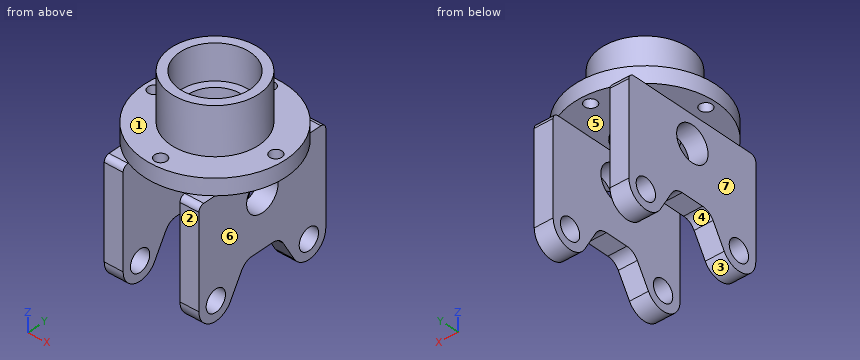
from build123d import *

# Parameters (mm, degrees)
SKETCH_1_R               = 52.5
EXTRUDE_1_DEPTH          = 12
SKETCH_2_R               = 32.5
EXTRUDE_2_DEPTH          = 35
SKETCH_3_R               = 26
CUT_EXTRUDE_1_DEPTH      = 26
SKETCH_4_R               = 20
CUT_EXTRUDE_2_DEPTH      = 21
SKETCH_5_R               = 8
SKETCH_5_R_2             = 13
EXTRUDE_3_DEPTH          = 35
SKETCH_6_W               = 42
SKETCH_6_H               = 101.243911614
CUT_EXTRUDE_3_DEPTH      = 153.922365925
SKETCH_7_R               = 4.5
CUT_EXTRUDE_4_DEPTH      = 114.615579918
PATTERN_CIRCULAR_1_COUNT = 4


with BuildPart() as part:
    # 草图1 → 凸台-拉伸1 (new body)
    with BuildSketch(Plane.XY):
        Circle(SKETCH_1_R)
    extrude(amount=-EXTRUDE_1_DEPTH)

    # 草图2 → 凸台-拉伸2 (add)
    with BuildSketch(Plane.XY):
        Circle(SKETCH_2_R)
    extrude(amount=EXTRUDE_2_DEPTH)

    # 草图3 → 切除-拉伸1 (cut)
    with BuildSketch(Plane.XY.offset(35)):
        Circle(SKETCH_3_R)
    extrude(amount=-CUT_EXTRUDE_1_DEPTH, mode=Mode.SUBTRACT)

    # 草图4 → 切除-拉伸2 (cut)
    with BuildSketch(Plane.XY.offset(9)):
        Circle(SKETCH_4_R)
    extrude(amount=-CUT_EXTRUDE_2_DEPTH, mode=Mode.SUBTRACT)

    # 草图5 → 凸台-拉伸3 (add, symmetric)
    with BuildSketch(Plane(origin=(0, 0, 0), x_dir=(0, 0, -1), z_dir=(1, 0, 0))):
        with BuildLine():
            Line((84, -52.5), (16, -52.5))
            ThreePointArc((16, -52.5), (13.171572875, -51.328427125), (12, -48.5))
            Line((12, -48.5), (12, 48.5))
            ThreePointArc((12, 48.5), (13.171572875, 51.328427125), (16, 52.5))
            Line((16, 52.5), (84, 52.5))
            ThreePointArc((84, 52.5), (97.522961568, 42.123466631), (91, 26.375644347))
            Line((91, 26.375644347), (75, 17.13804004))
            ThreePointArc((75, 17.13804004), (71.339745962, 13.477786002), (70, 8.477786002))
            Line((70, 8.477786002), (70, -8.477786002))
            ThreePointArc((70, -8.477786002), (71.339745962, -13.477786002), (75, -17.13804004))
            Line((75, -17.13804004), (91, -26.375644347))
            ThreePointArc((91, -26.375644347), (97.522961568, -42.123466631), (84, -52.5))
        make_face()
        with Locations((84, 38.5)):
            Circle(SKETCH_5_R, mode=Mode.SUBTRACT)
        with Locations((84, -38.5)):
            Circle(SKETCH_5_R, mode=Mode.SUBTRACT)
        with Locations((32, 0)):
            Circle(SKETCH_5_R_2, mode=Mode.SUBTRACT)
    extrude(amount=EXTRUDE_3_DEPTH, both=True)

    # 草图6 → 切除-拉伸3 (cut, through all)
    with BuildSketch(Plane.XZ.offset(52.5)):
        with Locations((0, -62.621955807)):
            Rectangle(SKETCH_6_W, SKETCH_6_H)
    extrude(amount=-CUT_EXTRUDE_3_DEPTH, mode=Mode.SUBTRACT)

    # 草图7 → 切除-拉伸4 (cut, through all)
    with BuildSketch(Plane(origin=(0, 0, -12), x_dir=(-1, 0, 0), z_dir=(0, 0, -1))):
        with Locations((-45, 0)):
            Circle(SKETCH_7_R)
    cut_extrude_4 = extrude(amount=-CUT_EXTRUDE_4_DEPTH, mode=Mode.SUBTRACT)

    # 阵列(圆周)1: 切除-拉伸4 ×4 about axis
    pattern_circular_1_axis = Axis((0, 0, 0), (0, 0, 1))
    for i in range(1, PATTERN_CIRCULAR_1_COUNT):
        add(cut_extrude_4.rotate(pattern_circular_1_axis, i * 360 / PATTERN_CIRCULAR_1_COUNT), mode=Mode.SUBTRACT)


solid = part.part
Build history of the part. All positions in model axes, mm. Face numbers are marked on the shaded views. A direction names the side the tool comes from. Give positions to 0.01 mm unless a question says otherwise; leave off trailing zeros. Write each loop counter-clockwise with the first axis right and the second up, starting at its lowest first coordinate (ties: lowest second). Pieces come first, ordered by that corner, then holes. Notation, with made-up numbers: (2.5, -25.75) - (21.5, -25.75) arc R34 ccw to (21.5, 4.25) - close; hole circle Ø4 at (55.25, 79). An arc over 180 degrees is marked (long way). Use one line per item in the form item = value. Start each with the question number.
1. Band-saw the part on C-C on y = 43. Write the cut outline in (x, z), plus the area to 3 significant figures.
2. 3-axis set-ups, long thin cutter, end or side, ignore diameter. For the marked faces 4, 5, 6 and 7: which of +Z, -Z, +X, -X, +Y, -Y reach the whole face in a straight line?
3. Band-saw the part on D-D on x = -45. Write the cut outline in (y, z).
4. Two-plate mould, pull along Y, no slides. Class the marked faces 1, 2 and 3: released by +Y, released by -Y, zero draft, split by the parting line, or undercut.
5. Drop flat-ended pins along their axis: pin 1 Ø1 at (x, y) = (40, -16.5) entering from +Z; pin 2 Ø8 at (x, y) = (-19.5, -21) entering from -Z; pin 3 Ø7 at (x, y) = (-26.5, -1) entering from -Z; pin 4 Ø12 at (x, z) = (19.5, -80.5) entering from -Y. Give the stop position or say it passes through.
6. Band-saw the part on B-B on x = 0. Write the cut outline in (y, z), plus the area to 3 significant figures.
7. Band-saw the part on A-A on z = -32. Write the cut outline in (x, y).
8. Probe line 1 (Y direction, x = 0, z = 23.75); line 2 (Z direction, x = -28, y = 1); line 3 (Y direction, x = -31.5, z = -84). List the from-to ranges inside material, lowest first. Write a range as [from, to].
Conclusion:
q1.outline = (-35, -97.26) - (-21, -97.26) - (-21, -90.61) - (-35, -90.61) - close; (-35, -77.39) - (-21, -77.39) - (-21, -12) - (-4.03, -12) - (-4.03, 0) - (-30.12, 0) - (-30.12, -12) - (-35, -12) - close; (4.03, -12) - (21, -12) - (21, -77.39) - (35, -77.39) - (35, -12) - (30.12, -12) - (30.12, 0) - (4.03, 0) - close; (21, -97.26) - (35, -97.26) - (35, -90.61) - (21, -90.61) - close
q1.area = 2,640 mm²
q2.face_4 = -Z, +X, -X
q2.face_5 = -Z, +Y, -Y
q2.face_6 = -Z, +X, +Y, -Y
q2.face_7 = -Z, -X, +Y, -Y
q3.outline = (-27.04, -12) - (-4.5, -12) - (-4.5, 0) - (-27.04, 0) - close; (4.5, -12) - (27.04, -12) - (27.04, 0) - (4.5, 0) - close
q4.face_1 = zero draft
q4.face_2 = released by -Y
q4.face_3 = undercut
q5.pin_1 = 0
q5.pin_2 = -88.11
q5.pin_3 = -70
q5.pin_4 = -52.5
q6.outline = (-52.5, -12) - (-49.5, -12) - (-49.5, 0) - (-52.5, 0) - close; (-40.5, -12) - (-20, -12) - (-20, 9) - (-26, 9) - (-26, 35) - (-32.5, 35) - (-32.5, 0) - (-40.5, 0) - close; (20, -12) - (40.5, -12) - (40.5, 0) - (32.5, 0) - (32.5, 35) - (26, 35) - (26, 9) - (20, 9) - close; (49.5, -12) - (52.5, -12) - (52.5, 0) - (49.5, 0) - close
q6.area = 1,130 mm²
q7.outline = (-35, -52.5) - (-21, -52.5) - (-21, -13) - (-35, -13) - close; (-35, 13) - (-21, 13) - (-21, 52.5) - (-35, 52.5) - close; (21, -52.5) - (35, -52.5) - (35, -13) - (21, -13) - close; (21, 13) - (35, 13) - (35, 52.5) - (21, 52.5) - close
q8.line_1 = [-32.5, -26], [26, 32.5]
q8.line_2 = [-70, -44.96], [-19.04, 35]
q8.line_3 = [-52.5, -46.5], [-30.5, -22.33], [22.33, 30.5], [46.5, 52.5]
